Job drawing, mm, ordinate dimensions from the low corner. One solid piece. A direction names the side the tool comes from. Give positions to 0.01 mm unless a question says otherwise; leave off trailing zeros. Loops run counter-clockwise (first coordinate to the right, second up) from the corner with the lowest first, then second, coordinate; pieces in that order, holes last. Notation, with made-up numbers: M 3,37 L 25,37 A18 ccw 25,55 Z; hole C -19.75,75 d6. An arc over 180 degrees is marked long. One line per question, with ' | ' between items.
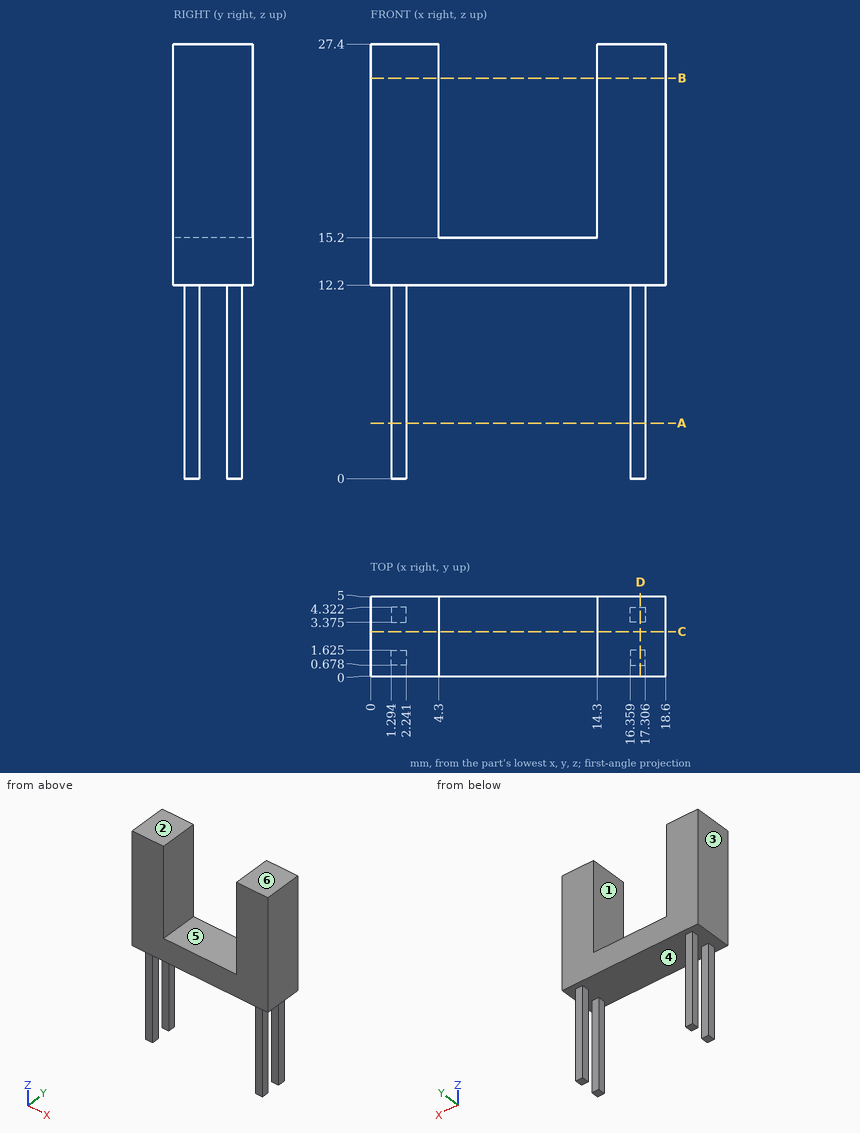
Item 1: Saw through at D-D on x = 17. Give the cut face in (y, z) (1 decimal).
Conclusion:
outline: M 0,12.2 L 0.7,12.2 L 0.7,0 L 1.6,0 L 1.6,12.2 L 3.4,12.2 L 3.4,0 L 4.3,0 L 4.3,12.2 L 5,12.2 L 5,27.4 L 0,27.4 Z
Item 2: Mould opens along X. For the marked faces 1, 2, 3 and 4 say: pulls with the +X half, pulls with the -X half, needs draft (parallel to the pull), parting line crosses it, or undercut.
Conclusion:
face 1: undercut | face 2: needs draft | face 3: pulls with the -X half | face 4: undercut
Item 3: 3-axis set-ups, long thin cutter, end or side, ignore diameter. For the marked faces 5 and 6: which of +Z, -Z, +X, -X, +Y, -Y reach the whole face in a straight line?
Conclusion:
face 5: +Z, +Y, -Y | face 6: +Z, +X, -X, +Y, -Y
Item 4: Saw through at A-A on z = 3.5. Give the cut face in (x, y) (1 decimal).
Conclusion:
outline: M 1.3,0.7 L 2.2,0.7 L 2.2,1.6 L 1.3,1.6 Z; M 1.3,3.4 L 2.2,3.4 L 2.2,4.3 L 1.3,4.3 Z; M 16.4,0.7 L 17.3,0.7 L 17.3,1.6 L 16.4,1.6 Z; M 16.4,3.4 L 17.3,3.4 L 17.3,4.3 L 16.4,4.3 Z
Item 5: Drop flat-ended pins along their axis: P1, Ø1, axis at x = 1.5, z = 7, coming from the -Y side; P2, Ø1, axis at y = 1, z = 7, coming from the -X side; P3, Ø1.5, axis at x = 8, y = 1.5, coming from the +Z side. Give the stop position or say it passes through.
Conclusion:
P1: y = 0.68 | P2: x = 1.29 | P3: z = 15.2
Item 6: Saw through at B-B on z = 25.25. Give the cut face in (x, y).
Conclusion:
outline: M 0,0 L 4.3,0 L 4.3,5 L 0,5 Z; M 14.3,0 L 18.6,0 L 18.6,5 L 14.3,5 Z
Item 7: Drill centre lines: line 1 along X through (y, z) = (3.35, 19.75); line 2 along X through (y, z) = (3.8, 6.25); line 3 along Z through (x, y) = (2.5, 0.45). Where is each one in solid material? Low to high. Write a range as [from, to].
Conclusion:
line 1: [0, 4.3], [14.3, 18.6] | line 2: [1.29, 2.24], [16.36, 17.31] | line 3: [12.2, 27.4]
Item 8: Saw through at C-C on y = 2.8. Give the cut face in (x, z), and give its area (3 significant figures).
Conclusion:
outline: M 0,12.2 L 18.6,12.2 L 18.6,27.4 L 14.3,27.4 L 14.3,15.2 L 4.3,15.2 L 4.3,27.4 L 0,27.4 Z | area: 161 mm²
